Design review of the part built by this model. Coordinates are the model's own, in mm. A direction names the side the tool comes from. Give positions to 0.01 mm unless a question says otherwise; leave off trailing zeros. Order: outer loops, then holes, each group sorted by start corner. A loop starts at its lowest first (then second) coordinate and runs counter-clockwise, first axis right, second up.
```python
from build123d import *

# Parameters (mm, degrees)
EXTRUDE_1_DEPTH      = 12.7
CUT_EXTRUDE_1_REACH  = 17.534
SKETCH_3_W           = 2.5
SKETCH_3_H           = 1.2
EXTRUDE_2_DEPTH      = 2
EXTRUDE_2_DEPTH_BACK = 2
SKETCH_5_W           = 1.4
SKETCH_5_H           = 2
CUT_EXTRUDE_2_REACH  = 17.39
CHAMFER_1_SIZE       = 1
CHAMFER_2_SIZE       = 0.8


with BuildPart() as part:
    # 草图2 → 凸台-拉伸1 (new body)
    with BuildSketch(Plane(origin=(0, 0, 0), x_dir=(1, 0, 0), z_dir=(0, 1, 0))):
        with BuildLine():
            Line((0, 2), (6, 2))
            ThreePointArc((6, 2), (8, 0), (6, -2))
            Line((6, -2), (0, -2))
            ThreePointArc((0, -2), (-2, 0), (0, 2))
        make_face()
    extrude(amount=EXTRUDE_1_DEPTH)

    # 草图3 → 切除-拉伸1 (cut, up to next)
    with BuildSketch(Plane.XY.offset(2), mode=Mode.PRIVATE) as cut_extrude_1_sk1:
        with Locations((-0.75, 0.6)):
            Rectangle(SKETCH_3_W, SKETCH_3_H)
    cut_extrude_1_tool1 = extrude(cut_extrude_1_sk1.sketch, amount=-CUT_EXTRUDE_1_REACH, mode=Mode.PRIVATE) & part.part
    # 草图3 → 切除-拉伸1 (cut, up to next)
    with BuildSketch(Plane.XY.offset(2), mode=Mode.PRIVATE) as cut_extrude_1_sk2:
        with Locations((6.75, 0.6)):
            Rectangle(SKETCH_3_W, SKETCH_3_H)
    cut_extrude_1_tool2 = extrude(cut_extrude_1_sk2.sketch, amount=-CUT_EXTRUDE_1_REACH, mode=Mode.PRIVATE) & part.part
    add(cut_extrude_1_tool1.solids().sort_by_distance((-0.75, 0.6, 2))[0], mode=Mode.SUBTRACT)
    add(cut_extrude_1_tool2.solids().sort_by_distance((6.75, 0.6, 2))[0], mode=Mode.SUBTRACT)

    # 草图5 → 凸台-拉伸2 (add, two sides: drawn at the far end of the back side and taken through both)
    with BuildSketch(Plane.ZY.offset(-3).offset(-EXTRUDE_2_DEPTH_BACK)):
        Polygon((-2, 7), (-2.4, 7), (-2.4, 8), (-2, 8.4), align=None)
        Polygon((2, 8.4), (2, 7), (2.4, 7), (2.4, 8), align=None)
        with Locations((-2.7, 2.2)):
            Rectangle(SKETCH_5_W, SKETCH_5_H)
        with Locations((2.7, 2.2)):
            Rectangle(SKETCH_5_W, SKETCH_5_H)
    extrude(amount=EXTRUDE_2_DEPTH + EXTRUDE_2_DEPTH_BACK)

    # 草图6 → 切除-拉伸2 (cut, up to next)
    with BuildSketch(Plane(origin=(0, 12.7, 0), x_dir=(1, 0, 0), z_dir=(0, 1, 0)), mode=Mode.PRIVATE) as cut_extrude_2_sk1:
        with BuildLine():
            Line((1.2, 2.4), (1, 2.4))
            Line((1, 2.4), (1, 2.236067977))
            ThreePointArc((1, 2.236067977), (1.098232815, 2.320189986), (1.2, 2.4))
        make_face()
    cut_extrude_2_tool1 = extrude(cut_extrude_2_sk1.sketch, amount=-CUT_EXTRUDE_2_REACH, mode=Mode.PRIVATE) & part.part
    # 草图6 → 切除-拉伸2 (cut, up to next)
    with BuildSketch(Plane(origin=(0, 12.7, 0), x_dir=(1, 0, 0), z_dir=(0, 1, 0)), mode=Mode.PRIVATE) as cut_extrude_2_sk2:
        with BuildLine():
            Line((4.8, -2.4), (5, -2.4))
            Line((5, -2.4), (5, -2.236067977))
            ThreePointArc((5, -2.236067977), (4.901767185, -2.320189986), (4.8, -2.4))
        make_face()
    cut_extrude_2_tool2 = extrude(cut_extrude_2_sk2.sketch, amount=-CUT_EXTRUDE_2_REACH, mode=Mode.PRIVATE) & part.part
    # 草图6 → 切除-拉伸2 (cut, up to next)
    with BuildSketch(Plane(origin=(0, 12.7, 0), x_dir=(1, 0, 0), z_dir=(0, 1, 0)), mode=Mode.PRIVATE) as cut_extrude_2_sk3:
        with BuildLine():
            Line((5, 2.4), (4.8, 2.4))
            ThreePointArc((4.8, 2.4), (4.901767185, 2.320189986), (5, 2.236067977))
            Line((5, 2.236067977), (5, 2.4))
        make_face()
    cut_extrude_2_tool3 = extrude(cut_extrude_2_sk3.sketch, amount=-CUT_EXTRUDE_2_REACH, mode=Mode.PRIVATE) & part.part
    # 草图6 → 切除-拉伸2 (cut, up to next)
    with BuildSketch(Plane(origin=(0, 12.7, 0), x_dir=(1, 0, 0), z_dir=(0, 1, 0)), mode=Mode.PRIVATE) as cut_extrude_2_sk4:
        with BuildLine():
            Line((1, -2.236067977), (1, -2.4))
            Line((1, -2.4), (1.2, -2.4))
            ThreePointArc((1.2, -2.4), (1.098232815, -2.320189986), (1, -2.236067977))
        make_face()
    cut_extrude_2_tool4 = extrude(cut_extrude_2_sk4.sketch, amount=-CUT_EXTRUDE_2_REACH, mode=Mode.PRIVATE) & part.part
    add(cut_extrude_2_tool1.solids().sort_by_distance((1.065681, 12.7, -2.346155))[0], mode=Mode.SUBTRACT)
    add(cut_extrude_2_tool2.solids().sort_by_distance((4.934319, 12.7, 2.346155))[0], mode=Mode.SUBTRACT)
    add(cut_extrude_2_tool3.solids().sort_by_distance((4.934319, 12.7, -2.346155))[0], mode=Mode.SUBTRACT)
    add(cut_extrude_2_tool4.solids().sort_by_distance((1.065681, 12.7, 2.346155))[0], mode=Mode.SUBTRACT)

    # 倒角1
    chamfer_1_edges = [part.edges().sort_by_distance(p)[0] for p in [
        (3, 1.2, -3.4),
        (3, 1.2, 3.4),
    ]]
    chamfer(chamfer_1_edges, length=CHAMFER_1_SIZE)

    # 倒角2
    chamfer_2_edges = [part.edges().sort_by_distance(p)[0] for p in [
        (8, 12.7, 0),
        (3, 12.7, -2),
        (-2, 12.7, 0),
        (3, 12.7, 2),
    ]]
    chamfer(chamfer_2_edges, length=CHAMFER_2_SIZE)


solid = part.part
```
1. Take a section at B-B (y = 3). State the section outline as (x, z) points, then the cut area to 3 significant figures.
Recorded:
outline: (0, -2) - (1, -2) - (1, -3.4) - (5, -3.4) - (5, -2) - (6, -2) arc R2 ccw to (6, 2) - (5, 2) - (5, 3.4) - (1, 3.4) - (1, 2) - (0, 2) arc R2 ccw to start
area: 47.8 mm2
2. For line 1 along Z through (x, y) = (0.5, 6); line 2 along Y through (x, z) = (6.25, 0); line 3 along Z through (x, y) = (1.5, 7.25), list the stretches that pass through material, from the lowest coordinate up.
Recorded:
line 1: z = -2 to 2
line 2: y = 1.2 to 12.7
line 3: z = -2.4 to 2.4
3. Draft analysis for pull direction Y (two halves, no side actions). For faces 1 (the face through (7.34, 12.56, -0.03)), 2 (the face through (3, 6, 2)), 3 (the face through (3, 3, 3.4)), state which applies: pulls with the +Y half, pulls with the -Y half, needs draft (parallel to the pull), parting line crosses it, or undercut.
Recorded:
face 1: pulls with the +Y half
face 2: undercut
face 3: needs draft
4. Machinability: for faces 4 (the face through (0.5, 1, 0)), 5 (the face through (5, 2.4, 2.7)), 6 (the face through (5, 2.4, -2.7)), 7 (the face through (1, 2.4, 2.7)), which of the approach directions +Z, -Z, +X, -X, +Y, -Y give a long, thin tool a straight path to every point of the face, cutting with its end or side? Answer none if there is none.
Recorded:
face 4: +Z, -Z, -X, -Y
face 5: +Z, +X, +Y, -Y
face 6: -Z, +X, +Y, -Y
face 7: +Z, -X, +Y, -Y
5. For pin 1 (0.7 mm diameter, centred on x = 3.5, z = 2.5, fed in from +Y); pin 2 (3 mm diameter, centred on x = 0, y = 4.5, fed in from +Z); pin 3 (0.7 mm diameter, centred on x = 4, z = -3, fed in from +Y), all flat-tipped, find the tip position at first contact; note any pin that passes through.
Recorded:
pin 1: stops at y = 8.25
pin 2: stops at z = 2
pin 3: stops at y = 3.2
6. Take a section at A-A (z = 0). State the section outline as (x, y) points, then the cut area to 3 significant figures.
Recorded:
outline: (-2, 1.2) - (0.5, 1.2) - (0.5, 0) - (5.5, 0) - (5.5, 1.2) - (8, 1.2) - (8, 11.9) - (7.2, 12.7) - (-1.2, 12.7) - (-2, 11.9) - close
area: 120 mm2
7. Take a section at D-D (y = 9.5). State the section outline as (x, z) points, then the cut area to 3 significant figures.
Recorded:
outline: (0, -2) - (6, -2) arc R2 ccw to (6, 2) - (0, 2) arc R2 ccw to start
area: 36.6 mm2
8. Take a section at C-C (z = 3). State the section outline as (x, y) points.
Recorded:
outline: (1, 1.8) - (5, 1.8) - (5, 3.2) - (1, 3.2) - close
